Job drawing, mm, ordinate dimensions from the low corner. One solid piece. A direction names the side the tool comes from. Coordinates: 2 decimals unless noted, no trailing zeros. Order: outer loops, then holes, each group sorted by start corner. A loop starts at its lowest first (then second) coordinate and runs counter-clockwise, first axis right, second up. Notation, with made-up numbers: (72, -38.75) -> (98, -38.75) arc R7 ccw to (98, -33.75) -> close; hole circle Ø11 at (83.5, -32.5). An arc over 180 degrees is marked (long way). Use CSV: the item, a comma, the result in double quotes. Start each with the question number.
(1) Cut at D-D on y = 3.5. Write the cut outline in (x, z), plus the area to 3 significant figures.
(2) Cut at C-C on x = 10. Write the cut outline in (y, z), plus the area to 3 significant figures.
(3) Probe L1, parallel to Z at x = 52, y = 17; L2, parallel to Y at x = 42.5, z = 46.5. List the from-to ranges inside material, lowest first.
(4) Cut at B-B on z = 30. Write the cut outline in (x, y).
(5) Cut at A-A on y = 15. Write the cut outline in (x, z), plus the area to 3 significant figures.
(6) Pin check, flat tips, straight feed: pin 1 Ø3 at (x, y) = (18.5, 29) entering from -Z; pin 2 Ø4 at (y, z) = (9, 14) entering from +X; pin 3 Ø3 at (x, z) = (41.5, 24) entering from +Y. Stop position of each tip, or through.
(7) Tool access for the marked faces 1, 2, 3 and 4: list every direction of +Z, -Z, +X, -X, +Y, -Y with a clear straight run to the whole face (end or side of a thin tool).
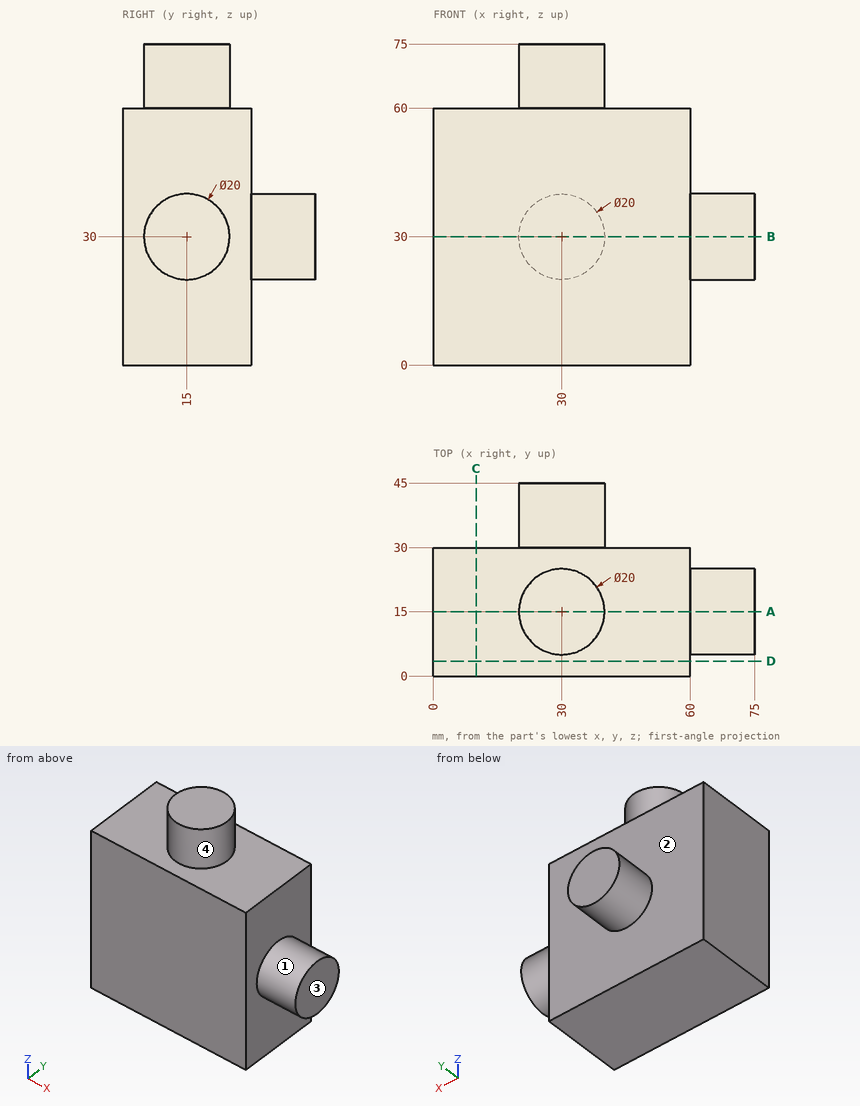
Outcome:
1,outline,"(0, 0) -> (60, 0) -> (60, 60) -> (0, 60) -> close"
1,area,"3,600 mm2"
2,outline,"(0, 0) -> (30, 0) -> (30, 60) -> (0, 60) -> close"
2,area,"1,800 mm2"
3,L1,"0 to 60"
3,L2,"0 to 30"
4,outline,"(0, 0) -> (60, 0) -> (60, 5) -> (75, 5) -> (75, 25) -> (60, 25) -> (60, 30) -> (40, 30) -> (40, 45) -> (20, 45) -> (20, 30) -> (0, 30) -> close"
5,outline,"(0, 0) -> (60, 0) -> (60, 20) -> (75, 20) -> (75, 40) -> (60, 40) -> (60, 60) -> (40, 60) -> (40, 75) -> (20, 75) -> (20, 60) -> (0, 60) -> close"
5,area,"4,200 mm2"
6,pin 1,"z = 0"
6,pin 2,"x = 60"
6,pin 3,"y = 30"
7,face 1,"+X"
7,face 2,"+Y"
7,face 3,"+Z, -Z, +X, +Y, -Y"
7,face 4,"+Z"
